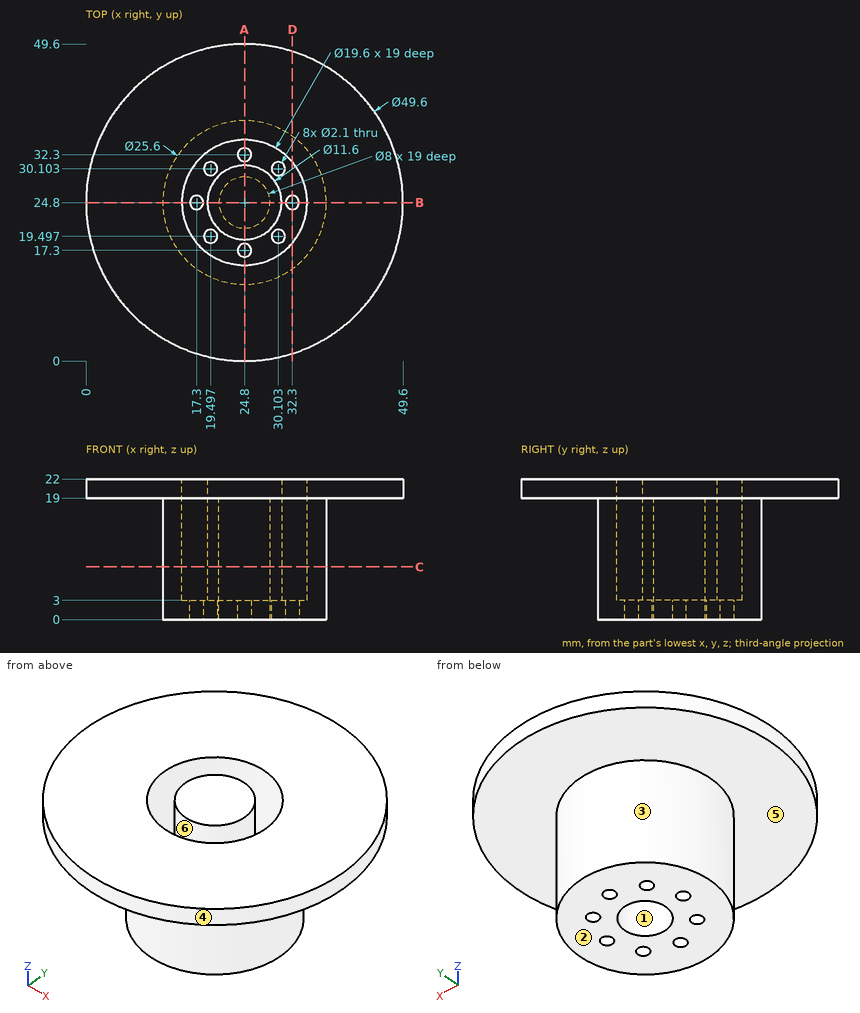
Geometry check sheet. Reference: drawing and pictorial views, mm from the part's lowest x, y, z. A direction names the side the tool comes from. Coordinates: 2 decimals unless noted, no trailing zeros. Write each loop counter-clockwise with the first axis right and the second up, starting at its lowest first coordinate (ties: lowest second). Pieces come first, ordered by that corner, then holes. Notation, with made-up numbers: (-33.5, 36.5) -> (16.5, 36.5) arc R18 cw to (16.5, 54.5) -> close; hole circle Ø4 at (48, 12.25). An arc over 180 degrees is marked (long way). One line per question, with ' | ' between items.
1. Draft check along X on the marked faces 1, 2 and 3. Enter one of: +X half, -X half, draft (parallel to the pull), parting line (faces both ways), or undercut.
Answers:
face 1: undercut | face 2: draft | face 3: parting line
2. Cross-section at D-D on x = 32.3. Record the cut outline in (y, z).
Answers:
outline: (1.16, 19) -> (14.43, 19) -> (14.43, 0) -> (23.75, 0) -> (23.75, 3) -> (18.49, 3) -> (18.49, 22) -> (1.16, 22) -> close; (25.85, 0) -> (35.17, 0) -> (35.17, 19) -> (48.44, 19) -> (48.44, 22) -> (31.11, 22) -> (31.11, 3) -> (25.85, 3) -> close
3. Depth check by flat-ended pin: pin 1 Ø3 at (y, z) = (14.5, 8) entering from -X (1 decimal); pin 2 Ø1.5 at (x, z) = (12.5, 12.5) entering from -Y (1 decimal); pin 3 Ø12 at (y, z) = (16.5, 13.5) entering from +X. Enter the tip coordinate at first touch or a pass-through.
Answers:
pin 1: stops at x = 15.5 | pin 2: stops at y = 19.3 | pin 3: stops at x = 48.89
4. Set-up check for the marked faces 4, 5 and 6: record each of +Z, -Z, +X, -X, +Y, -Y from which the full face is reachable in a straight line by a thin tool's end or side.
Answers:
face 4: +Z, -Z | face 5: -Z | face 6: +Z
5. Thickness scan on probe 1 along Y at (x, z) = (22.5, 11) (1 decimal); probe 2 along Z at (x, y) = (47.5, 22.5); probe 3 along Y at (x, z) = (18, 9.75) (1 decimal). Record the ranges inside material, lowest first. Write a range as from..to.
Answers:
probe 1: y = 12.2..15.3, 19.5..21.5, 28.1..30.1, 34.3..37.4 | probe 2: z = 19..22 | probe 3: y = 14..17.7, 31.9..35.6
6. Cross-section at A-A on x = 24.8. Record the cut outline in (y, z).
Answers:
outline: (0, 19) -> (12, 19) -> (12, 0) -> (16.25, 0) -> (16.25, 3) -> (15, 3) -> (15, 22) -> (0, 22) -> close; (18.35, 0) -> (20.8, 0) -> (20.8, 19) -> (28.8, 19) -> (28.8, 0) -> (31.25, 0) -> (31.25, 3) -> (30.6, 3) -> (30.6, 22) -> (19, 22) -> (19, 3) -> (18.35, 3) -> close; (33.35, 0) -> (37.6, 0) -> (37.6, 19) -> (49.6, 19) -> (49.6, 22) -> (34.6, 22) -> (34.6, 3) -> (33.35, 3) -> close
7. Cross-section at C-C on z = 8.25. Record the cut outline in (x, y).
Answers:
outline: circle Ø25.6 at (24.8, 24.8); circle Ø11.6 at (24.8, 24.8); hole circle Ø19.6 at (24.8, 24.8); hole circle Ø8 at (24.8, 24.8)
